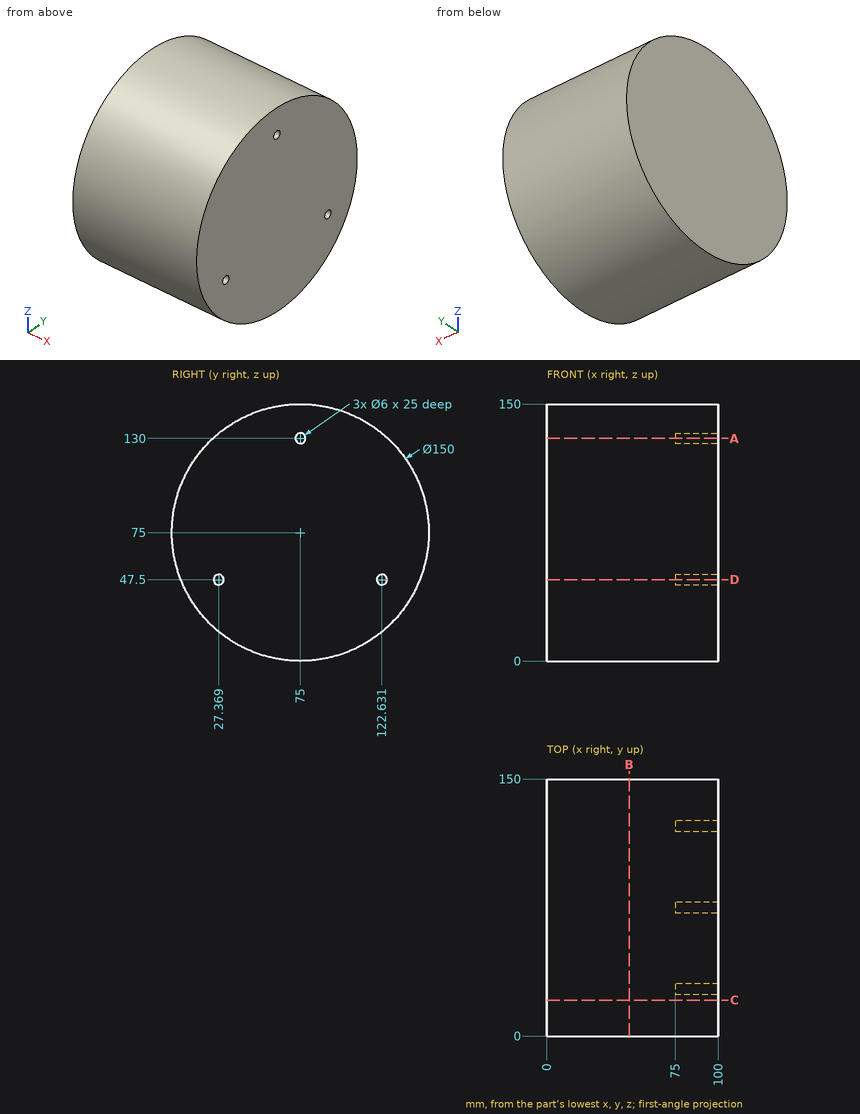
Print and shaded views of the part. All mm, measured from the part's lowest x, y and z. Give positions to 0.01 mm unless a question says otherwise; leave off trailing zeros. Loops run counter-clockwise (first coordinate to the right, second up) from the corner with the lowest first, then second, coordinate; pieces in that order, holes last. Notation, with made-up numbers: (64.25, -9) -> (110.25, -9) arc R8 ccw to (110.25, -3) -> close; hole circle Ø2 at (-39.5, -23). An arc over 180 degrees is marked (long way). Use a Markdown table: item, result.
1. Slice it at B-B (x = 48). List the corners of the cut face in (y, z).
Check result:
| item | result |
|---|---|
| outline | circle Ø150 at (75, 75) |
2. Flat gauge pins, fed straight in: pin 1 (8 mm diameter, centred on x = 38.5, y = 118.5, fed in from +Z) (1 decimal); pin 2 (5 mm diameter, centred on x = 27.5, y = 132.5, fed in from +Z); pin 3 (1.8 mm diameter, centred on y = 122.5, z = 48, fed in from +X). Where does each tip first touch, or does it go through?
Check result:
| item | result |
|---|---|
| pin 1 | stops at z = 138.8 |
| pin 2 | stops at z = 125.99 |
| pin 3 | stops at x = 75 |
3. Slice it at A-A (z = 130). List the corners of the cut face in (x, y), plus the area to 3 significant figures.
Check result:
| item | result |
|---|---|
| outline | (0, 24.01) -> (100, 24.01) -> (100, 72) -> (75, 72) -> (75, 78) -> (100, 78) -> (100, 125.99) -> (0, 125.99) -> close |
| area | 10,000 mm^2 |
4. Slice it at C-C (y = 21). List the corners of the cut face in (x, z), plus the area to 3 significant figures.
Check result:
| item | result |
|---|---|
| outline | (0, 22.95) -> (100, 22.95) -> (100, 127.05) -> (0, 127.05) -> close |
| area | 10,400 mm^2 |
5. Slice it at D-D (z = 47.5). List the corners of the cut face in (x, y).
Check result:
| item | result |
|---|---|
| outline | (0, 5.22) -> (100, 5.22) -> (100, 24.37) -> (75, 24.37) -> (75, 30.37) -> (100, 30.37) -> (100, 119.63) -> (75, 119.63) -> (75, 125.63) -> (100, 125.63) -> (100, 144.78) -> (0, 144.78) -> close |
6. Wall check: L1, parallel to Y at x = 85, z = 47; L2, parallel to Z at x = 92, y = 75; L3, parallel to Y at x = 45, z = 76. Give the ranges that are in metal, low to high. Write a range as [from, to].
Check result:
| item | result |
|---|---|
| L1 | y = [5.42, 24.41], [30.33, 119.67], [125.59, 144.58] |
| L2 | z = [0, 127], [133, 150] |
| L3 | y = [0.01, 149.99] |
